The drawing under review shows one solid part. Ordinate dimensions are in mm from its lowest x, y, z. A direction names the side the tool comes from. Round coordinates to 2 decimals unless told otherwise and drop trailing zeros. Write each loop counter-clockwise with the first axis right and the second up, starting at its lowest first coordinate (ties: lowest second). Pieces come first, ordered by that corner, then holes. Notation, with made-up numbers: M 63.5,51 L 67.5,51 A20 cw 67.5,70 Z; hole C 1.25,5.25 d7. An arc over 180 degrees is marked long. One line per item, written item: value. Start each with the question number.
1) Take a section at A-A, the plane y = 15.24. Write out the cut boundary in (x, z) (1 decimal), and give its area (3 significant figures).
2) Wall thickness on probe 1 along X at (y, z) = (15, 57); probe 2 along Z at (x, y) = (46, 21.5); probe 3 along X at (y, z) = (11.5, 64): over which ranges is each line inside the solid? List them lowest first.
3) For P1, Ø6, axis at y = 26, z = 81, coming from the -X side; P2, Ø1.5, axis at y = 11, z = 89, coming from the -X side (1 decimal); P3, Ø1.5, axis at y = 3.5, z = 30.5, coming from the +X side (1 decimal); P4, Ø2.5, axis at x = 78, y = 3.5, coming from the -Z side, all flat-tipped, find the tip position at first contact; note any pin that passes through.
4) Mouldability with a two-part tool opening along Z and no side actions: class the marked faces 1, 2 and 3 as +Z half, -Z half, draft (parallel to the pull), parting line (faces both ways), or undercut.
5) Take a section at D-D, the plane z = 68. Write out the cut boundary in (x, y), and give its area (3 significant figures).
6) Take a section at C-C, the plane z = 45. Write out the cut boundary in (x, y).
7) Tool access review of the marked faces 4, 5 and 6: name each direction out of +Z, -Z, +X, -X, +Y, -Y from which nothing blocks a thin tool from reaching the whole face with its end or side.
8) Take a section at B-B, the plane x = 12.7. Write out the cut boundary in (y, z).
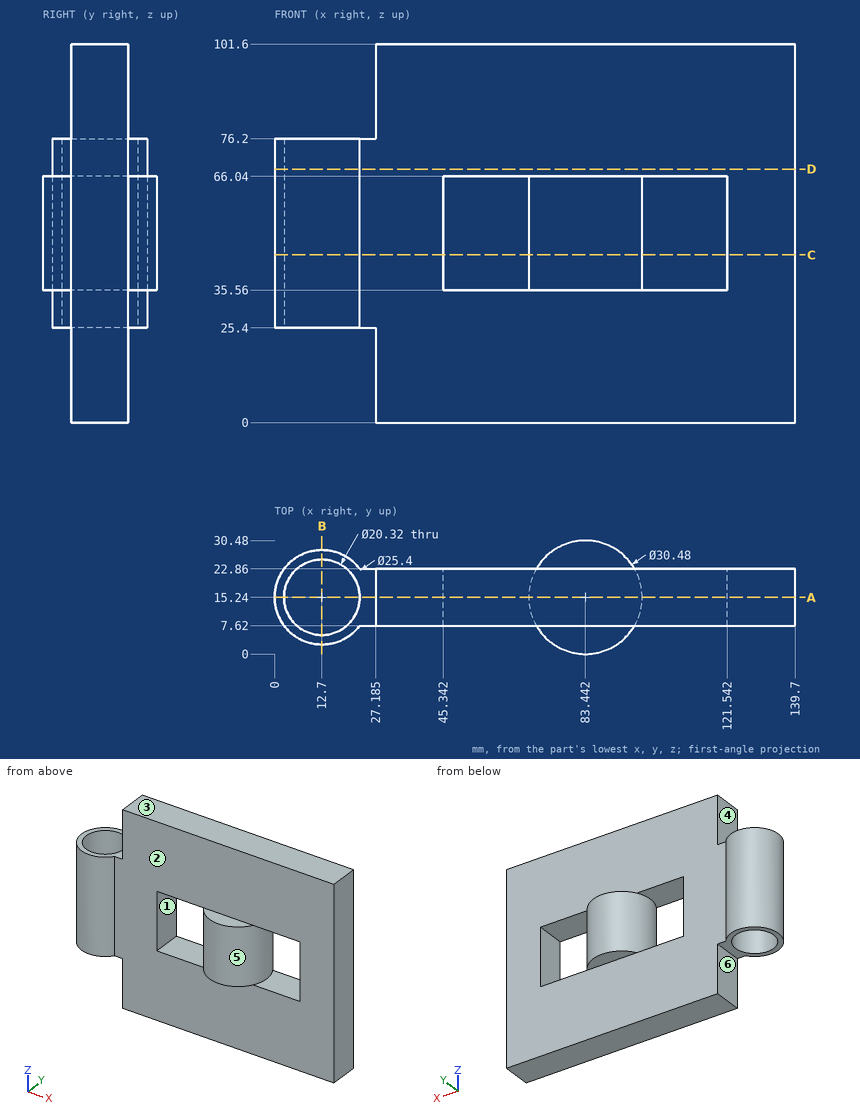
Checked values:
1. outline: M 0,25.4 L 2.5,25.4 L 2.5,76.2 L 0,76.2 Z; M 22.9,25.4 L 27.2,25.4 L 27.2,0 L 139.7,0 L 139.7,101.6 L 27.2,101.6 L 27.2,76.2 L 22.9,76.2 Z; hole M 45.3,35.6 L 68.2,35.6 L 68.2,66 L 45.3,66 Z; hole M 98.7,35.6 L 121.5,35.6 L 121.5,66 L 98.7,66 Z
1. area: 10,400 mm2
2. probe 1: x = 0 to 2.54, 22.86 to 45.34, 68.2 to 98.68, 121.54 to 139.7
2. probe 2: z = 0 to 35.56, 66.04 to 101.6
2. probe 3: x = 0.56 to 3.25, 22.15 to 45.34, 68.67 to 98.22, 121.54 to 139.7
3. P1: passes through
3. P2: stops at x = 27.2
3. P3: stops at x = 19.1
3. P4: stops at z = 35.56
4. face 1: undercut
4. face 2: draft
4. face 3: +Z half
5. outline: M 22.86,7.62 L 139.7,7.62 L 139.7,22.86 L 22.86,22.86 A12.7 ccw long Z; hole C 12.7,15.24 d20.32
5. area: 1,940 mm2
6. outline: M 22.86,7.62 L 45.34,7.62 L 45.34,22.86 L 22.86,22.86 A12.7 ccw long Z; C 83.44,15.24 d30.48; M 121.54,7.62 L 139.7,7.62 L 139.7,22.86 L 121.54,22.86 Z; hole C 12.7,15.24 d20.32
7. face 4: +Z, -X, +Y, -Y
7. face 5: none
7. face 6: -Z, -X, +Y, -Y
8. outline: M 2.54,25.4 L 5.08,25.4 L 5.08,76.2 L 2.54,76.2 Z; M 25.4,25.4 L 27.94,25.4 L 27.94,76.2 L 25.4,76.2 Z
